Autodesk Inventor part; units mm, degrees
ref_plane "YZ Plane" through (0, 0, 0) normal (1, 0, 0) x (0, 1, 0)
ref_plane "XZ Plane" through (0, 0, 0) normal (0, 1, 0) x (-1, 0, 0)
ref_plane "XY Plane" through (0, 0, 0) normal (0, 0, 1) x (1, 0, 0)
sketch "Sketch9" plane through (0, 0, 0) normal (0, 1, 0) x (-1, 0, 0)
  circle A0 centre (0, 0) radius 12.6365
  dimension "d53" = 25.273
extrude "Extrusion6" add sketch "Sketch9" along normal mid plane 2.54
sketch "Sketch15" plane through (0, 1.27, 0) normal (0, 1, 0) x (1, 0, 0)
  line L0 (7.9923, 0) -> (3.9961, -6.9215)
  line L1 (3.9961, -6.9215) -> (-3.9961, -6.9215)
  line L2 (-3.9961, -6.9215) -> (-7.9923, 0)
  line L3 (-7.9923, 0) -> (-3.9961, 6.9215)
  line L4 (-3.9961, 6.9215) -> (3.9961, 6.9215)
  line L5 (3.9961, 6.9215) -> (7.9923, 0)
  point P0 (0, 0)
  point P1 (0, 0)
  dimension "d82" = 13.843
extrude "Extrusion11" cut sketch "Sketch15" against normal through all
chamfer "Chamfer7" distance 0.7937 angle 45 6 edges at (-5.9942, 1.27, -3.4607) (-5.9942, 1.27, 3.4608) (0, 1.27, 6.9215) (5.9942, 1.27, 3.4607) (5.9942, 1.27, -3.4608) (0, 1.27, -6.9215)
equation "\"d82\" = hexDiameter"
equation "\"holeForString\" = stringDiameter + clearanceForString"
equation "\"stringDiameter\" = 3.048"
equation "\"clearanceForString\" = 2.032"
equation "\"spoolHeightWithoutSpacer\" = 69.85"
equation "\"hexShaftDiameter\" = 12.7"
equation "\"clearanceForHexShaft\" = 1.143"
equation "\"hexDiameter\" = hexShaftDiameter + clearanceForHexShaft"
equation "\"supportChannels\" = 3.81"
equation "\"spoolInteriorDiameter\" = 38.1"
equation "\"spoolInteriroRadius\" = 0.5 * spoolInteriorDiameter"
equation "\"spoolExteriorDiameter\" = 88.9"
equation "\"spoolExteriorRadius\" = 0.5 * spoolExteriorDiameter"
equation "\"spoolFiletRadius\" = 0.5 * supportChannels"
equation "\"holeCenter\" = 0.25 * spoolHeightWithoutSpacer - 0.75 * supportChannels"
equation "\"hexHoleChamfer\" = 1.5875"
equation "\"stringHoleCenterFromHexShaft\" = 0.5 * hexDiameter + 0.5 * holeForString"
equation "\"textCircleDiameter\" = 0.75 * spoolExteriorDiameter"
equation "\"textHeight\" = 6.096"
equation "\"textDepth\" = 1.27"
equation "\"stringHoleChamfer\" = 4.7625"
equation "\"spoolTotalHeight\" = 76.2"
equation "\"spaceHeight\" = spoolTotalHeight - spoolHeightWithoutSpacer"
equation "\"spacerDiameter\" = 24.13"
properties part number "spacerForEndV08" material "PC/ABS Plastic"
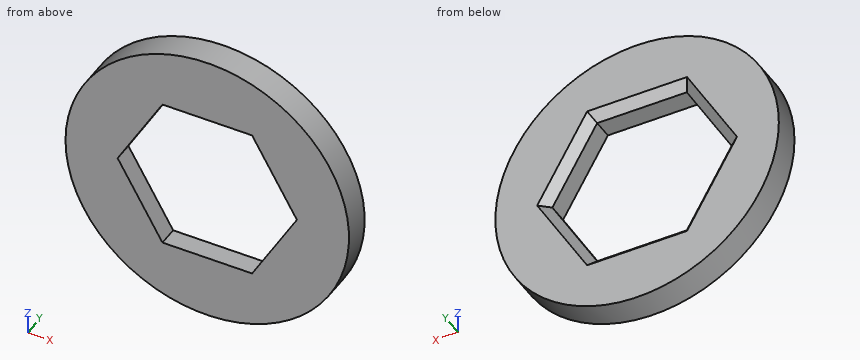
Part model, mm, in its own coordinate system. Give positions to 0.01 mm unless a question says otherwise; leave off trailing zeros. Loops run counter-clockwise (first coordinate to the right, second up) from the corner with the lowest first, then second, coordinate; pieces in that order, holes last. Notation, with made-up numbers: M 5,54 L 26,54 A6 ccw 26,59 Z; hole C 22,-35 d6. An arc over 180 degrees is marked long. Put each result on its own line as item: value. Start each with the question number.
1) Flat gauge pins, fed straight in: pin 1 (1 mm diameter, centred on y = -0.5, z = -6.5, fed in from -X); pin 2 (0.5 mm diameter, centred on x = 1, y = 0, fed in from -Z). Where does each tip first touch, or does it go through?
2) Saw through at D-D (x = -9.75). List the corners of the cut face in (y, z), then the cut area to 3 significant figures.
3) Probe probe 1 along X at (y, z) = (0.15, 5.25); probe 2 along Z at (x, y) = (-5.75, -0.2); probe 3 along Z at (x, y) = (-3.5, 1.1). List the from-to ranges inside material, lowest first.
4) Saw through at A-A (x = 0). List the corners of the cut face in (y, z).
5) Saw through at C-C (z = -4.25). List the corners of the cut face in (x, y) (3 decimals).
6) Saw through at B-B (y = -0.9). List the corners of the cut face in (x, z).
Numbers:
1. pin 1: x = -11.12
1. pin 2: z = -12.61
2. outline: M -1.27,-8.04 L 1.27,-8.04 L 1.27,8.04 L -1.27,8.04 Z
2. area: 40.8 mm^2
3. probe 1: -11.49 to -4.96, 4.96 to 11.49
3. probe 2: -11.25 to -3.88, 3.88 to 11.25
3. probe 3: -12.14 to -7.55, 7.55 to 12.14
4. outline: M -1.27,-12.64 L 1.27,-12.64 L 1.27,-7.72 L 0.48,-6.92 L -1.27,-6.92 Z; M -1.27,6.92 L 0.48,6.92 L 1.27,7.72 L 1.27,12.64 L -1.27,12.64 Z
5. outline: M -11.9,-1.27 L -5.539,-1.27 L -5.539,0.476 L -6.455,1.27 L -11.9,1.27 Z; M 5.539,-1.27 L 11.9,-1.27 L 11.9,1.27 L 6.455,1.27 L 5.539,0.476 Z
6. outline: C 0,0 d25.27; hole M -7.99,0 L -4,-6.92 L 4,-6.92 L 7.99,0 L 4,6.92 L -4,6.92 Z
